Check sheet for the modelled part. Datum: model origin and axes. Units: mm. A direction names the side the tool comes from. Round coordinates to 2 decimals unless told otherwise and drop trailing zeros. Write each loop counter-clockwise with the first axis right and the second up, starting at its lowest first coordinate (ties: lowest second). Pieces come first, ordered by that corner, then holes. Notation, with made-up numbers: (44.25, 45.5) -> (97.25, 45.5) arc R18 cw to (97.25, 68.5) -> close; hole circle Ø10 at (82, 77). An arc over 180 degrees is marked (long way). One line per item, written item: value.
from build123d import *

# Parameters (mm, degrees)
ESQUISSE1_W             = 5
ESQUISSE1_H             = 58
BOSS_EXTRU_1_DEPTH      = 18
ESQUISSE2_W             = 3
ESQUISSE2_H             = 47.75
BOSS_EXTRU_2_DEPTH      = 10
ESQUISSE3_R             = 1.625
ENL_V_MAT_EXTRU_1_DEPTH = 4
ENL_V_MAT_EXTRU_2_DEPTH = 59


with BuildPart() as part:
    # Esquisse1 → Boss.-Extru.1 (new body)
    with BuildSketch(Plane.XY):
        with Locations((2.5, -29)):
            Rectangle(ESQUISSE1_W, ESQUISSE1_H)
    extrude(amount=BOSS_EXTRU_1_DEPTH)

    # Esquisse2 → Boss.-Extru.2 (add)
    with BuildSketch(Plane.ZY):
        with Locations((1.5, -34.125)):
            Rectangle(ESQUISSE2_W, ESQUISSE2_H)
    extrude(amount=BOSS_EXTRU_2_DEPTH)

    # Esquisse3 → Enlèv. mat.-Extru.1 (cut, through all)
    with BuildSketch(Plane.XY.offset(3)):
        with Locations((-5, -15)):
            Circle(ESQUISSE3_R)
        with Locations((-5, -43)):
            Circle(ESQUISSE3_R)
    extrude(amount=-ENL_V_MAT_EXTRU_1_DEPTH, mode=Mode.SUBTRACT)

    # Esquisse4 → Enlèv. mat.-Extru.2 (cut, through all)
    with BuildSketch(Plane.XZ.offset(58)):
        Polygon((0, 18), (0, 17.75), (5, 18), align=None)
    extrude(amount=-ENL_V_MAT_EXTRU_2_DEPTH, mode=Mode.SUBTRACT)


solid = part.part
Item 1: Thickness scan on line 1 (Y direction, x = -5, z = 0.85) (3 decimals); line 2 (X direction, y = -23.5, z = 15.5); line 3 (Z direction, x = -6.25, y = -56). Record the ranges inside material, lowest first.
Answer:
line 1: y = -58 to -44.625, -41.375 to -16.625, -13.375 to -10.25
line 2: x = 0 to 5
line 3: z = 0 to 3
Item 2: Mould release check, pull along X, two halves, no side actions. Record for faces 1 (the flat face through (-2, -36, 0)), 2 (the flat face through (2.465, -29.406, 17.873)), 3 (the cylindrical face through (-5.352, -16.586, 1.521)): pulls with the +X half, pulls with the -X half, needs draft (parallel to the pull), parting line crosses it, or undercut.
Answer:
face 1: needs draft
face 2: pulls with the -X half
face 3: undercut
Item 3: Sectioned sample at D-D on y = -52.5. Enter the section's corners in (x, z), and give its area (3 significant figures).
Answer:
outline: (-10, 0) -> (5, 0) -> (5, 18) -> (0, 17.75) -> (0, 3) -> (-10, 3) -> close
area: 119 mm^2
Item 4: Sectioned sample at C-C on y = -43. Enter the section's corners in (x, z) (3 decimals), and give its area (3 significant figures).
Answer:
outline: (-10, 0) -> (-6.625, 0) -> (-6.625, 3) -> (-10, 3) -> close; (-3.375, 0) -> (5, 0) -> (5, 18) -> (0, 17.75) -> (0, 3) -> (-3.375, 3) -> close
area: 110 mm^2
Item 5: Depth check by flat-ended pin: P1, Ø1.5, axis at x = -2.5, z = 1, coming from the +Y side; P2, Ø3, axis at x = -2.5, z = 14.5, coming from the +Y side; P3, Ø9, axis at y = -27.5, z = 12, coming from the -X side; P4, Ø4, axis at x = -8, y = -38.5, coming from the +Z side. Enter the tip coordinate at first touch or a pass-through.
Answer:
P1: stops at y = -10.25
P2: passes through
P3: stops at x = 0
P4: stops at z = 3
Item 6: Sectioned sample at A-A on z = 1.75. Enter the section's corners in (x, y) (3 decimals), and give its area (3 significant figures).
Answer:
outline: (-10, -58) -> (5, -58) -> (5, 0) -> (0, 0) -> (0, -10.25) -> (-10, -10.25) -> close; hole circle Ø3.25 at (-5, -43); hole circle Ø3.25 at (-5, -15)
area: 751 mm^2
Item 7: Tool access check on faces 4 (the flat face through (-10, -34, 1)), 5 (the flat face through (-5, -10.25, 1)), 6 (the flat face through (-5, -34, 3)). Record the directions out of +Z, -Z, +X, -X, +Y, -Y that give a thin tool (end or side, any length) a straight path to the whole face; none if there is none.
Answer:
face 4: +Z, -Z, -X, +Y, -Y
face 5: +Z, -Z, -X, +Y
face 6: +Z, -X, +Y, -Y
Item 8: Sectioned sample at B-B on x = -5. Enter the section's corners in (y, z) (3 decimals), and give its area (3 significant figures).
Answer:
outline: (-58, 0) -> (-44.625, 0) -> (-44.625, 3) -> (-58, 3) -> close; (-41.375, 0) -> (-16.625, 0) -> (-16.625, 3) -> (-41.375, 3) -> close; (-13.375, 0) -> (-10.25, 0) -> (-10.25, 3) -> (-13.375, 3) -> close
area: 124 mm^2
